The model under review builds one solid part; all positions refer to its coordinate system, in mm. Round coordinates to 2 decimals unless told otherwise and drop trailing zeros. Order: outer loops, then holes, each group sorted by start corner. A loop starts at its lowest first (then second) coordinate and runs counter-clockwise, first axis right, second up.
1) Clearance check with flat-ended pins moving along their axes: P1, Ø2, axis at y = 4, z = 1.5, coming from the -X side; P2, Ø1.2, axis at x = -16, z = 0, coming from the +Y side. State where each tip first meets the part, or that it passes through.
2) Consider section B-B (x = 16). Give the boundary of the cut face in (y, z), then the cut area to 3 significant figures.
3) Consider section C-C (y = 6.75). Give the boundary of the cut face in (x, z).
4) To check wall thickness, follow L1, parallel to Z at x = 34, y = 1.75; L2, parallel to X at y = 5.75, z = 1.25; L3, parallel to Z at x = -34.5, y = 4. State the ranges of each line that lie inside material, in increasing order.
5) Consider section A-A (z = 0). Give the boundary of the cut face in (x, y), then the cut area to 3 significant figures.
from build123d import *

# Parameters (mm, degrees)
SKETCH_1_R      = 0.75
SKETCH_1_R_2    = 2
EXTRUDE_1_DEPTH = 8


with BuildPart() as part:
    # 草圖1 → 填料-伸長1 (new body)
    with BuildSketch(Plane(origin=(0, 0, 0), x_dir=(1, 0, 0), z_dir=(0, 1, 0))):
        with BuildLine():
            Line((-0.414012206, -4), (25, -4))
            Line((25, -4), (34, -4))
            ThreePointArc((34, -4), (38, 0), (34, 4))
            Line((34, 4), (25, 4))
            Line((25, 4), (-0.414012206, 4))
            Line((-0.414012206, 4), (-34, 4))
            ThreePointArc((-34, 4), (-38, 0), (-34, -4))
            Line((-34, -4), (-0.414012206, -4))
        make_face()
        with Locations(Location((34, 0, 0), (0, 0, 270))):
            Circle(SKETCH_1_R, mode=Mode.SUBTRACT)
        with Locations(Location((-34, 0, 0), (0, 0, 270))):
            Circle(SKETCH_1_R, mode=Mode.SUBTRACT)
        with Locations(Location((-25, 0, 0), (0, 0, 270))):
            Circle(SKETCH_1_R_2, mode=Mode.SUBTRACT)
        with Locations(Location((25, 0, 0), (0, 0, 270))):
            Circle(SKETCH_1_R_2, mode=Mode.SUBTRACT)
        with Locations(Location((-16, 0, 0), (0, 0, 270))):
            Circle(SKETCH_1_R, mode=Mode.SUBTRACT)
        with Locations(Location((16, 0, 0), (0, 0, 270))):
            Circle(SKETCH_1_R, mode=Mode.SUBTRACT)
    extrude(amount=EXTRUDE_1_DEPTH)


solid = part.part
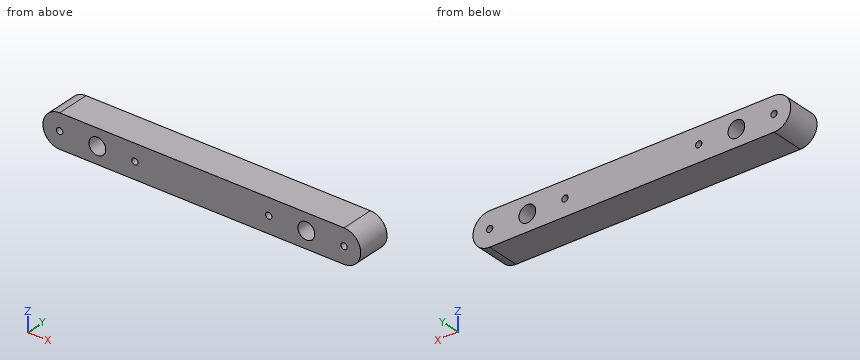
Answer below:
1. P1: stops at x = -37.97
1. P2: passes through
2. outline: (0, -4) - (8, -4) - (8, -0.75) - (0, -0.75) - close; (0, 0.75) - (8, 0.75) - (8, 4) - (0, 4) - close
2. area: 52.0 mm2
3. outline: (-34, -4) - (34, -4) arc R4 ccw to (34, 4) - (-34, 4) arc R4 ccw to start; hole circle Ø1.5 at (-34, 0); hole circle Ø4 at (-25, 0); hole circle Ø1.5 at (-16, 0); hole circle Ø1.5 at (16, 0); hole circle Ø4 at (25, 0); hole circle Ø1.5 at (34, 0)
4. L1: z = -4 to -0.75, 0.75 to 4
4. L2: x = -37.8 to -26.56, -23.44 to 23.44, 26.56 to 37.8
4. L3: z = -3.97 to -0.56, 0.56 to 3.97
5. outline: (-38, 0) - (-34.75, 0) - (-34.75, 8) - (-38, 8) - close; (-33.25, 0) - (-27, 0) - (-27, 8) - (-33.25, 8) - close; (-23, 0) - (-16.75, 0) - (-16.75, 8) - (-23, 8) - close; (-15.25, 0) - (15.25, 0) - (15.25, 8) - (-15.25, 8) - close; (16.75, 0) - (23, 0) - (23, 8) - (16.75, 8) - close; (27, 0) - (33.25, 0) - (33.25, 8) - (27, 8) - close; (34.75, 0) - (38, 0) - (38, 8) - (34.75, 8) - close
5. area: 496 mm2
